Autodesk Inventor part; units mm, degrees
ref_plane "YZ Plane" through (0, 0, 0) normal (1, 0, 0) x (0, 1, 0)
ref_plane "XZ Plane" through (0, 0, 0) normal (0, 1, 0) x (-1, 0, 0)
ref_plane "XY Plane" through (0, 0, 0) normal (0, 0, 1) x (1, 0, 0)
sketch "Sketch1" plane through (0, 0, 0) normal (0, 0, 1) x (1, 0, 0)
  arc A0 (5.1615, 6.0904) -> (2.4461, 7.62) centre (2.4461, 4.445) ccw construction
  line L0 (2.4461, 7.62) -> (-28.575, 7.62) construction
  arc A1 (-28.575, 7.62) -> (-31.75, 4.445) centre (-28.575, 4.445) ccw construction
  line L1 (-31.75, 4.445) -> (-31.75, -0.344) construction
  arc A2 (-31.75, -0.344) -> (-31.6418, -1.1658) centre (-28.575, -0.344) ccw construction
  line L2 (-29.5221, -9.0768) -> (-31.6418, -1.1658) construction
  arc A3 (-29.5221, -9.0768) -> (-26.4553, -11.43) centre (-26.4553, -8.255) ccw construction
  line L3 (-26.4553, -11.43) -> (9.525, -11.43) construction
  arc A4 (9.525, -11.43) -> (12.7, -8.255) centre (9.525, -8.255) ccw
  line L4 (12.7, -8.255) -> (12.7, -7.2369)
  arc A5 (12.7, -7.2369) -> (12.2404, -5.5915) centre (9.525, -7.2369) ccw
  line L5 (5.1615, 6.0904) -> (12.2404, -5.5915) construction
  line L6 (4.7625, 12.7) -> (-16.1925, 12.7)
  line L7 (-16.1925, 12.7) -> (-16.1925, -11.43)
  line L8 (-16.1925, -11.43) -> (4.7625, -11.43)
  line L9 (4.7625, -11.43) -> (4.7625, 12.7) construction
  line L10 (4.7625, -11.43) -> (9.525, -11.43)
  line L11 (12.2404, -5.5915) -> (1.1563, 12.7)
  point P0 (0, 0)
  dimension "d0" = 20.955
  dimension "d1" = 24.13
  dimension "d2" = 4.7625
extrude "Extrusion1" add sketch "Sketch1" along normal blind 22.225
sketch "Sketch2" plane through (0, 0, 22.225) normal (0, 0, 1) x (1, 0, 0)
  circle A0 centre (0, 0) radius 2.5019 construction
  circle A1 centre (-6.35, 0) radius 2.5527 construction
  circle A2 centre (-19.05, 0) radius 2.5527 construction
  circle A3 centre (-25.4, 0) radius 2.5019 construction
  point P0 (0, 0)
hole "Hole1" at (0, 0, 22.225) direction (0, 0, -1) diameter 5.0038 end through all
hole "Hole2" at (-6.35, 0, 22.225) at (-19.05, 0, 22.225) direction (0, 0, -1) diameter 4.9784 end through all
sketch "Sketch3" plane through (-16.1925, 12.7, 0) normal (0, 1, 0) x (1, 0, 0)
  line L0 (16.1925, -14.2875) -> (8.255, -14.2875) construction
  line L1 (-46.1199, -6.35) -> (861.9301, -6.35) construction
  line L2 (0, 0) -> (0, -22.225) construction
  point P0 (16.1925, 0)
  dimension "d19" = 7.9375
  dimension "d21" = 7.9375
  dimension "d31" = 8.255
hole "Hole3" at (-7.9375, 12.7, 14.2875) direction (0, -1, 0) diameter 3.9624 depth 13.6144 tip angle 118
fillet "Fillet1" radius 9.525 1 edges at (-16.1925, -11.43, 11.1125)
fillet "Fillet2" radius 3.175 2 edges at (-16.1925, 12.7, 11.1125) (1.1563, 12.7, 11.1125)
properties part number "BEARING,MOUNT,SIDE,ELEVATOR"
Model file for the job. Use its own axes, mm. A direction names the side the tool comes from. Give positions to 0.01 mm unless a question says otherwise; leave off trailing zeros. Order: outer loops, then holes, each group sorted by start corner. A loop starts at its lowest first (then second) coordinate and runs counter-clockwise, first axis right, second up. Notation, with made-up numbers: M 79,64 L 130,64 A8 ccw 130,77 Z; hole C 27.25,58.25 d7. An arc over 180 degrees is marked long. Put each result on its own line as item: value. Start each with the question number.
(1) Band-saw the part on A-A on x = -1.75. Give the cut face in (y, z) (3 decimals), then the cut area to 3 significant figures.
(2) Pin check, flat tips, straight feed: pin 1 Ø3 at (x, z) = (7.5, 3.5) entering from +Y; pin 2 Ø4.5 at (x, z) = (-7.94, 14.29) entering from -Y; pin 3 Ø10 at (x, z) = (8, 8.5) entering from +Y. Stop position of each tip, or through.
(3) Drill centre lines: L1, parallel to X at y = 0, z = 14; L2, parallel to X at y = -2.25, z = 4; L3, parallel to Y at x = 0, z = 16.75. Where is each one in solid material? Low to high. Write a range as [from, to].
(4) Tool access for faces 1 (the face through (-9.9, 7.31, 14.03)), 2 (the face through (12.58, -6.37, 10.96)): list every direction of +Z, -Z, +X, -X, +Y, -Y with a clear straight run to the whole face (end or side of a thin tool).
(5) Band-saw the part on D-D on y = 7.75. Give the cut face in (x, z) (1 decimal), then the cut area to 3 significant figures.
(6) Band-saw the part on C-C on y = 0.75. Give the cut face in (x, z) (1 decimal).
(7) Band-saw the part on B-B on z = 11.25. Count the separate pieces of the cut face and the enclosed holes in it, then the cut area to 3 significant figures.
(8) Pull direction X, two halves, no side cores. Call faces 3 (the face through (12.7, -8, 11)), 4 (the face through (-13.476, -8.566, 11.268)), 5 (the face through (-8.703, -1.634, 14.117)): released by +X, released by -X, zero draft, split by the parting line, or undercut.
Results below:
1. outline: M -11.43,0 L -1.788,0 L -1.788,22.225 L -11.43,22.225 Z; M 1.788,0 L 12.7,0 L 12.7,22.225 L 1.788,22.225 Z
1. area: 457 mm2
2. pin 1: stops at y = 4.71
2. pin 2: stops at y = -11.43
2. pin 3: stops at y = 9.66
3. L1: x = [-16.19, -9.9], [-3.86, -2.5], [2.5, 8.85]
3. L2: x = [-16.19, -7.41], [-5.29, -1.09], [1.09, 10.22]
3. L3: y = [-11.43, -2.5], [2.5, 12.64]
4. face 1: +Y
4. face 2: +Z, -Z, +X, +Y
5. outline: M -16.2,0 L 4.2,0 L 4.2,22.2 L -16.2,22.2 Z; hole C -7.9,14.3 d4
5. area: 440 mm2
6. outline: M -16.2,0 L -8.7,0 L -8.7,12.5 A2 cw -8.7,16.1 L -8.7,22.2 L -16.2,22.2 Z; M -4,0 L -2.4,0 L -2.4,22.2 L -4,22.2 Z; M 2.4,0 L 8.4,0 L 8.4,22.2 L 2.4,22.2 Z
7. separate pieces: 1
7. enclosed holes: 2
7. area: 524 mm2
8. face 3: released by +X
8. face 4: released by -X
8. face 5: undercut
